from build123d import *

# Parameters (mm, degrees)
BASE_EXTRUDE_DEPTH  = 20
SKETCH3_R           = 40
BOSS_EXTRUDE1_DEPTH = 35
SKETCH4_R           = 35
CUT_EXTRUDE1_DEPTH  = 30
CUT_EXTRUDE2_DEPTH  = 10
SKETCH6_R           = 10
CUT_EXTRUDE3_DEPTH  = 121.415945788
CUT_EXTRUDE5_DEPTH  = 120.268604419


with BuildPart() as part:
    # Sketch1 → Base-Extrude (new body)
    with BuildSketch(Plane.XY):
        with BuildLine():
            Line((90, -20), (-60, -20))
            Line((-60, -20), (-60, 20))
            Line((-60, 20), (90, 20))
            ThreePointArc((90, 20), (97.071067812, 17.071067812), (100, 10))
            Line((100, 10), (100, -10))
            ThreePointArc((100, -10), (97.071067812, -17.071067812), (90, -20))
        make_face()
    extrude(amount=-BASE_EXTRUDE_DEPTH)

    # Sketch3 → Boss-Extrude1 (add)
    with BuildSketch(Plane.XY):
        with Locations((-60, 20)):
            Circle(SKETCH3_R)
    extrude(amount=-BOSS_EXTRUDE1_DEPTH)

    # Sketch4 → Cut-Extrude1 (cut)
    with BuildSketch(Plane(origin=(0, 0, -35), x_dir=(-1, 0, 0), z_dir=(0, 0, -1))):
        with Locations((60, 20)):
            Circle(SKETCH4_R)
    extrude(amount=-CUT_EXTRUDE1_DEPTH, mode=Mode.SUBTRACT)

    # Sketch5 → Cut-Extrude2 (cut)
    with BuildSketch(Plane(origin=(0, 0, -20), x_dir=(-1, 0, 0), z_dir=(0, 0, -1))):
        with BuildLine():
            Line((-90, -15), (20, -15))
            ThreePointArc((20, -15), (24.472135955, -12.236067977), (24, -7))
            ThreePointArc((24, -7), (18.955698609, 1.551007525), (15.90918463, 11))
            ThreePointArc((15.90918463, 11), (14.172482805, 13.872983346), (11.010205144, 15))
            Line((11.010205144, 15), (-90, 15))
            ThreePointArc((-90, 15), (-93.535533906, 13.535533906), (-95, 10))
            Line((-95, 10), (-95, -10))
            ThreePointArc((-95, -10), (-93.535533906, -13.535533906), (-90, -15))
        make_face()
    extrude(amount=-CUT_EXTRUDE2_DEPTH, mode=Mode.SUBTRACT)

    # Sketch6 → Cut-Extrude3 (cut, through all)
    with BuildSketch(Plane(origin=(0, 0, -5), x_dir=(-1, 0, 0), z_dir=(0, 0, -1))):
        with Locations((60, 20)):
            Circle(SKETCH6_R)
    extrude(amount=-CUT_EXTRUDE3_DEPTH, mode=Mode.SUBTRACT)

    # Sketch8 → Cut-Extrude5 (cut, through all)
    with BuildSketch(Plane(origin=(0, 0, -10), x_dir=(-1, 0, 0), z_dir=(0, 0, -1))):
        with BuildLine():
            Line((-83, -8), (9.275252588, -8))
            ThreePointArc((9.275252588, -8), (10.981793154, -7.042937821), (11.055068287, -5.087719298))
            ThreePointArc((11.055068287, -5.087719298), (8.543194297, 0.578436035), (6.684776274, 6.49122807))
            ThreePointArc((6.684776274, 6.49122807), (5.974361642, 7.578362465), (4.746040866, 8))
            Line((4.746040866, 8), (-83, 8))
            ThreePointArc((-83, 8), (-84.414213562, 7.414213562), (-85, 6))
            Line((-85, 6), (-85, -6))
            ThreePointArc((-85, -6), (-84.414213562, -7.414213562), (-83, -8))
        make_face()
    extrude(amount=-CUT_EXTRUDE5_DEPTH, mode=Mode.SUBTRACT)


solid = part.part
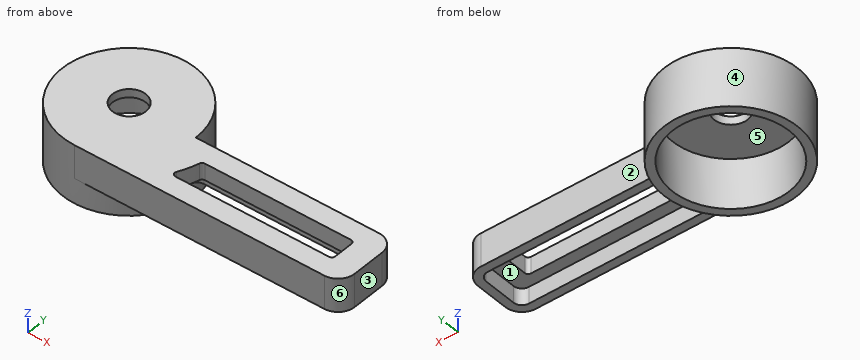
Geometry check sheet. Reference: the model listing, model coordinates, mm. Face numbers are marked on the shaded views. A direction names the side the tool comes from. Coordinates: 2 decimals unless noted, no trailing zeros. Order: outer loops, then holes, each group sorted by start corner. A loop starts at its lowest first (then second) coordinate and runs counter-clockwise, first axis right, second up. Notation, with made-up numbers: M -21.5,-15.75 L 14.5,-15.75 A35 cw 14.5,19.25 Z; hole C -3,3.5 d9. An arc over 180 degrees is marked long. Use CSV: the item, a comma, the result in double quotes.
Item 1: Thickness scan on line 1 along Y through (x, z) = (15.5, -14); line 2 along Y through (x, z) = (-60, -25); line 3 along Z through (x, y) = (-74.5, -5.5). Record the ranges inside material, lowest first.
Returned:
line 1,"y = -20 to -15, 15 to 20"
line 2,"y = -20 to -15, 55 to 60"
line 3,"z = -5 to 0"
Item 2: Cross-section at C-C on x = 87. Record the cut outline in (y, z).
Returned:
outline,"M -20,-20 L -15,-20 L -15,-10 L 15,-10 L 15,-20 L 20,-20 L 20,0 L -20,0 Z"
Item 3: Cross-section at D-D on y = 36.5. Record the cut outline in (x, z), then the cut area to 3 significant figures.
Returned:
outline,"M -96.44,-35 L -90.87,-35 L -90.87,-5 L -29.13,-5 L -29.13,-35 L -23.56,-35 L -23.56,0 L -96.44,0 Z"
area,"699 mm2"
Item 4: Gauge pin test, flat ends, axial feed: pin 1 Ø2 at (y, z) = (1, -22) entering from -X; pin 2 Ø1.5 at (x, y) = (3.5, 14) entering from -Z; pin 3 Ø6 at (x, z) = (-70.5, -26) entering from -Y; pin 4 Ø12 at (x, y) = (-60, 20) entering from -Z. Record the tip position at first contact, or that the pin passes through.
Returned:
pin 1,"stops at x = -95.72"
pin 2,"stops at z = -10"
pin 3,"stops at y = -19.29"
pin 4,"passes through"
Item 5: Tool access check on the marked faces 1, 2 and 3. Record the directions out of +Z, -Z, +X, -X, +Y, -Y that give a thin tool (end or side, any length) a straight path to the whole face; none if there is none.
Returned:
face 1,"-Z"
face 2,"+Z, -Z, +X, +Y"
face 3,"+Z, -Z, +X, +Y, -Y"
Item 6: Cross-section at B-B on z = -16. Record the cut outline in (x, y).
Returned:
outline,"M -60,-20 L 90,-20 A10 ccw 100,-10 L 100,10 A10 ccw 90,20 L -20,20 A40 ccw long Z; hole C -60,20 d70; hole M -24,-7 A5 ccw -20,-15 L 90,-15 A5 ccw 95,-10 L 95,10 A5 ccw 90,15 L -11.01,15 A5 ccw -15.91,11 A45 cw Z"
Item 7: Cross-section at A-A on x = 4. Record the cut outline in (y, z).
Returned:
outline,"M -20,-20 L -15,-20 L -15,-10 L -8,-10 L -8,0 L -20,0 Z; M 8,-10 L 15,-10 L 15,-20 L 20,-20 L 20,0 L 8,0 Z"
Item 8: Mould release check, pull along X, two halves, no side actions. Record for the marked faces 4, 5 and 6: pulls with the +X half, pulls with the -X half, needs draft (parallel to the pull), parting line crosses it, or undercut.
Returned:
face 4,"parting line crosses it"
face 5,"undercut"
face 6,"pulls with the +X half"
